Study the drawing (mm; zero at the part's minimum x, y, z) and answer. Round coordinates to 2 decimals unless told otherwise and drop trailing zeros. Write each loop counter-clockwise with the first axis right and the second up, starting at its lowest first coordinate (ties: lowest second). Pieces come first, ordered by that corner, then holes. Notation, with made-up numbers: (64, 5.5) - (116, 5.5) arc R17 ccw to (116, 25.5) - close; hole circle Ø3 at (35, 38.5). An arc over 180 degrees is marked (long way). Use one line per item in the form item = value. Start each with the question number.
1) Each of these flat-tipped pins is pushed along its axis until it touches: pin 1 (12 mm diameter, centred on x = 14.5, y = 19, fed in from +Z); pin 2 (8 mm diameter, centred on y = 54.5, z = 84, fed in from +X) (1 decimal). Where does it stop, or does it pass through?
2) The part is cut by section A-A, the plane y = 61.5. Give the vertices of the cut face in (x, z), plus the area to 3 significant figures.
3) The part is cut by section B-B, the plane x = 28.5. Give the vertices of the cut face in (y, z), plus the area to 3 significant figures.
4) The part is cut by section C-C, the plane z = 79. Give the vertices of the cut face in (x, y), plus the area to 3 significant figures.
5) Consider line 1 along Z through (x, y) = (6, 91) (1 decimal); line 2 along X through (y, z) = (9, 69) (1 decimal); line 3 along X through (y, z) = (66.5, 96) (1 decimal). Determine where each line is inside the solid, lowest interval first. Write a range as from..to.
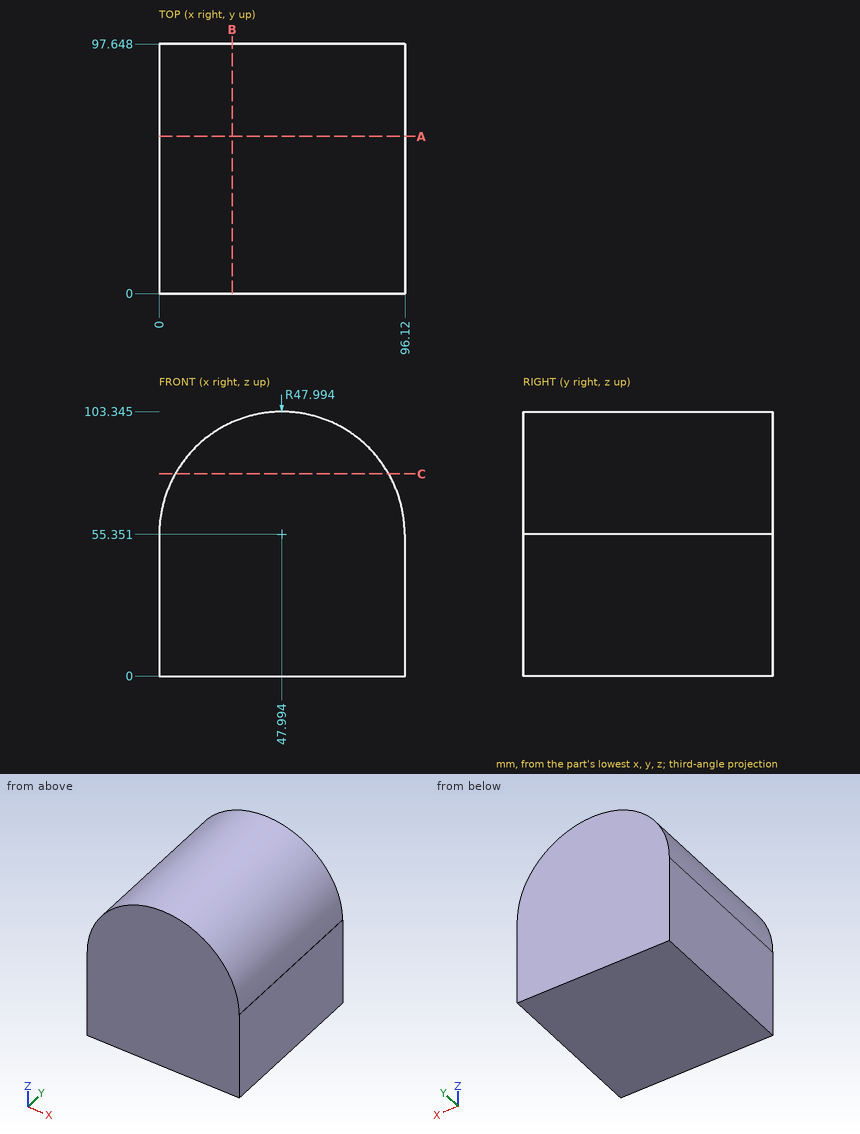
Geometry results:
q1.pin_1 = 94.69
q1.pin_2 = 89.2
q2.outline = (0, 0) - (96.12, 0) - (96.12, 55.35) - (95.99, 55.35) arc R47.99 ccw to (0, 55.35) - close
q2.area = 8,940 mm2
q3.outline = (0, 0) - (97.65, 0) - (97.65, 99.21) - (0, 99.21) - close
q3.area = 9,690 mm2
q4.outline = (6.23, 0) - (89.76, 0) - (89.76, 97.65) - (6.23, 97.65) - close
q4.area = 8,160 mm2
q5.line_1 = 0..78.6
q5.line_2 = 2..94
q5.line_3 = 22.5..73.5
